Build history of the part. All positions in model axes, mm. A direction names the side the tool comes from. Round coordinates to 2 decimals unless told otherwise and drop trailing zeros. Write each loop counter-clockwise with the first axis right and the second up, starting at its lowest first coordinate (ties: lowest second). Pieces come first, ordered by that corner, then holes. Notation, with made-up numbers: (22.25, -33) - (69.25, -33) arc R19 cw to (69.25, -10) - close; hole circle Ø9 at (18, -28). An arc over 180 degrees is marked (long way). One line per question, with ' | ' between items.
from build123d import *

# Parameters (mm, degrees)
SKETCH1_W          = 20
SKETCH1_H          = 27.8
BODY_DEPTH         = 6
BODY_DEPTH_BACK    = 6
SKETCH2_W          = 20
SKETCH2_H          = 1
CUTTHROUGH_DEPTH   = 13
RIBS_COUNT         = 10
RIBS_PITCH         = 1.8
SKETCH3_R          = 1.353942753
TOP_HOLES_DEPTH    = 13
SKETCH4_R          = 1.5
LOWERHOLE_DEPTH    = 6
SKETCH5_R          = 20
SKETCH5_R_2        = 10
CYLINDER_DEPTH     = 28.8
SKETCH6_R          = 4.3
CENTRE_ROD_DEPTH   = 23.8
SKETCH7_R          = 5.5
SKETCH7_R_2        = 4.9
UPPER_ROD_DEPTH    = 7.6
SKETCH7_2_R        = 4.9
UP_HOLE_DEPTH      = 7.6
SKETCH9_R          = 1.5
BOTTOM_HOLE_DEPTH  = 5
SKETCH10_R         = 3.5
CUT_EXTRUDE7_DEPTH = 21.2
FILLET1_R          = 1
FILLET2_R          = 1


with BuildPart() as part:
    # Sketch1 → body (new body, two sides)
    with BuildSketch(Plane.XY) as body_sk:
        Rectangle(SKETCH1_W, SKETCH1_H)
    extrude(amount=BODY_DEPTH)
    extrude(body_sk.sketch, amount=-BODY_DEPTH_BACK)

    # Sketch2 → cutThrough (cut, through all)
    with BuildSketch(Plane.XY.offset(6)):
        with Locations((0, -9.4)):
            Rectangle(SKETCH2_W, SKETCH2_H)
    cutthrough = extrude(amount=-CUTTHROUGH_DEPTH, mode=Mode.SUBTRACT)

    # ribs: cutThrough ×10
    with Locations(*[(0, i * RIBS_PITCH, 0) for i in range(1, RIBS_COUNT)]):
        add(cutthrough, mode=Mode.SUBTRACT)

    # Sketch3 → top holes (cut, through all)
    with BuildSketch(Plane.XY.offset(6)):
        with Locations((-7, 9.9)):
            Circle(SKETCH3_R)
    top_holes = extrude(amount=-TOP_HOLES_DEPTH, mode=Mode.SUBTRACT)

    # top hole R: top holes across plane
    add(top_holes.mirror(Plane(origin=(0, 0, 0), x_dir=(0, 0, 1), z_dir=(1, 0, 0))), mode=Mode.SUBTRACT)

    # Sketch4 → lowerHole (cut)
    with BuildSketch(Plane.XY.offset(6)):
        with Locations((0, -11.9)):
            Circle(SKETCH4_R)
    extrude(amount=-LOWERHOLE_DEPTH, mode=Mode.SUBTRACT)

    # Sketch5 → cylinder (cut, through all)
    with BuildSketch(Plane(origin=(0, 13.9, 0), x_dir=(1, 0, 0), z_dir=(0, 1, 0))):
        Circle(SKETCH5_R)
        Circle(SKETCH5_R_2, mode=Mode.SUBTRACT)
    extrude(amount=-CYLINDER_DEPTH, mode=Mode.SUBTRACT)

    # Sketch6 → centre rod (add)
    with BuildSketch(Plane(origin=(0, 13.9, 0), x_dir=(1, 0, 0), z_dir=(0, 1, 0))):
        Circle(SKETCH6_R)
    extrude(amount=-CENTRE_ROD_DEPTH)

    # Sketch7 → upper rod (add)
    with BuildSketch(Plane(origin=(0, 13.9, 0), x_dir=(1, 0, 0), z_dir=(0, 1, 0))):
        Circle(SKETCH7_R)
        Circle(SKETCH7_R_2, mode=Mode.SUBTRACT)
    extrude(amount=-UPPER_ROD_DEPTH)

    # Sketch7_2 → up hole (cut)
    with BuildSketch(Plane(origin=(0, 13.9, 0), x_dir=(1, 0, 0), z_dir=(0, 1, 0))):
        Circle(SKETCH7_2_R)
    extrude(amount=-UP_HOLE_DEPTH, mode=Mode.SUBTRACT)

    # Sketch9 → bottom hole (cut)
    with BuildSketch(Plane.XZ.offset(13.9)):
        with Locations((-7, -1.5)):
            Circle(SKETCH9_R)
    bottom_hole = extrude(amount=-BOTTOM_HOLE_DEPTH, mode=Mode.SUBTRACT)

    # bottom hole R: bottom hole across plane
    add(bottom_hole.mirror(Plane(origin=(0, 0, 0), x_dir=(0, 0, 1), z_dir=(1, 0, 0))), mode=Mode.SUBTRACT)

    # Sketch10 → Cut-Extrude7 (cut, through all)
    with BuildSketch(Plane(origin=(0, 6.3, 0), x_dir=(1, 0, 0), z_dir=(0, 1, 0))):
        Circle(SKETCH10_R)
    extrude(amount=-CUT_EXTRUDE7_DEPTH, mode=Mode.SUBTRACT)

    # Fillet1
    fillet1_edges = [part.edges().sort_by_distance(p)[0] for p in [
        (-4.9, 6.3, 0),
    ]]
    fillet(fillet1_edges, radius=FILLET1_R)

    # Fillet2
    fillet2_edges = [part.edges().sort_by_distance(p)[0] for p in [
        (-3.5, 6.3, 0),
    ]]
    fillet(fillet2_edges, radius=FILLET2_R)


solid = part.part
Q1. Saw through at C-C, the plane z = 2.75. State how many separate pieces and enclosed holes the cut face has, then the cut area to 3 significant figures.
Found:
separate pieces: 2 | enclosed holes: 2 | area: 251 mm^2
Q2. Saw through at B-B, the plane y = 9.9. List the corners of the cut face in (x, z), then the cut area to 3 significant figures.
Found:
outline: (-8.35, -5.5) - (-8.35, 5.5) arc R10 ccw to start; (-5.65, -6) - (5.65, -6) - (5.65, 6) - (-5.65, 6) - close; (8.35, -5.5) arc R10 ccw to (8.35, 5.5) - close; hole circle Ø9.8 at (0, 0) | area: 84.6 mm^2
Q3. Saw through at A-A, the plane y = -11.9. List the corners of the cut face in (x, z).
Found:
outline: (-8, -6) - (8, -6) arc R10 ccw to (8, 6) - (1.5, 6) - (1.5, 3.16) arc R3.5 cw (long way) to (-1.5, 3.16) - (-1.5, 6) - (-8, 6) arc R10 ccw to start; hole circle Ø3 at (-7, -1.5); hole circle Ø3 at (7, -1.5)
Q4. Drill centre lines: L1, parallel to Z at x = 7, y = -11.2; L2, parallel to X at y = 9.9, z = 0; L3, parallel to X at y = -8, z = 0. Where is each one in solid material? Low to high. Write a range as from..to.
Found:
L1: -6..-3, 0..6 | L2: -10..-8.35, -5.65..-4.9, 4.9..5.65, 8.35..10 | L3: -4.3..-3.5, 3.5..4.3
Q5. Drop flat-ended pins along their axis: pin 1 (6 mm diameter, centred on x = 1, z = 0.5, fed in from +Y); pin 2 (2 mm diameter, centred on y = -10, z = 1.5, fed in from +X); pin 3 (1 mm diameter, centred on x = -0.5, z = -4, fed in from +Y). Give the stop position or say it passes through.
Found:
pin 1: y = 6.32 | pin 2: x = 9.99 | pin 3: y = 6.52
Q6. Which spindle directions (+Z, -Z, +X, -X, +Y, -Y) get a long thin tool onto all of the face, cutting with end or side? Do faces 4 (the flat face through (0, 4, -6)), 5 (the cylindrical face through (-4.296, 5.007, -0.189)). Say none if no direction does.
Found:
face 4: -Z, +X, -X, +Y, -Y | face 5: none
Q7. Pull direction Y, two halves, no side cores. Call faces 1 (the flat face through (-5, 3.7, 0)), 2 (the flat face through (4.3, 13.9, -2.8)), 3 (the cylindrical face through (10, 2.3, 0.1)): +Y half, -Y half, draft (parallel to the pull), parting line (faces both ways), or undercut.
Found:
face 1: undercut | face 2: +Y half | face 3: draft
